Autodesk Inventor part; units mm, degrees
ref_plane "YZ Plane" through (0, 0, 0) normal (1, 0, 0) x (0, 1, 0)
ref_plane "XZ Plane" through (0, 0, 0) normal (0, 1, 0) x (-1, 0, 0)
ref_plane "XY Plane" through (0, 0, 0) normal (0, 0, 1) x (1, 0, 0)
sketch "Sketch1" plane through (0, 0, 0) normal (0, 0, 1) x (1, 0, 0)
  line L0 (0, 0) -> (160, 0)
  line L1 (160, 0) -> (160, 140)
  line L2 (160, 140) -> (0, 140)
  line L3 (0, 140) -> (0, 0)
  dimension "d0" = 160
  dimension "d1" = 140
extrude "Extrusion1" add sketch "Sketch1" along normal blind 3
fillet "Fillet1" radius 5 4 edges at (160, 140, 1.5) (0, 140, 1.5) (0, 0, 1.5) (160, 0, 1.5)
sketch "Sketch2" plane through (0, 0, 3) normal (0, 0, 1) x (1, 0, 0)
  arc A0 (155, 0) -> (160, 5) centre (155, 5) ccw
  line L0 (160, 5) -> (160, 135)
  arc A1 (160, 135) -> (155, 140) centre (155, 135) ccw
  line L1 (155, 140) -> (5, 140)
  arc A2 (5, 140) -> (0, 135) centre (5, 135) ccw
  line L2 (0, 135) -> (0, 5)
  arc A3 (0, 5) -> (5, 0) centre (5, 5) ccw
  line L3 (5, 0) -> (155, 0)
  line L4 (0, 0) -> (12.5, 0)
  line L5 (12.5, 0) -> (12.5, 12.5)
  line L6 (12.5, 12.5) -> (0, 12.5)
  line L7 (0, 12.5) -> (0, 0)
  circle A4 centre (12.5, 12.5) radius 1.5
  line L8 (80, 0) -> (80, 5)
  line L9 (0, 70) -> (5, 70)
  circle A5 centre (147.5, 12.5) radius 1.5
  circle A6 centre (12.5, 127.5) radius 1.5
  circle A7 centre (147.5, 127.5) radius 1.5
  dimension "d5" = 12.5
  dimension "d6" = 12.5
  dimension "d7" = 3
  dimension "d8" = 5
  dimension "d9" = 5
extrude "Extrusion2" cut sketch "Sketch2" against normal through all contours A4 L6 L5 | L5 L6 A4 | A5 | A6 | A7
fillet "Fillet2" radius 3 8 edges at (1.4645, 138.5355, 0) (0, 70, 0) (1.4645, 1.4645, 0) (80, 0, 0) (158.5355, 1.4645, 0) (160, 70, 0) (158.5355, 138.5355, 0) (80, 140, 0)
sketch "Sketch3" plane through (0, 0, 0) normal (0, 0, -1) x (-1, 0, 0)
  line L0 (-155, 140) -> (-5, 140)
  line L1 (-5, 0) -> (-155, 0)
  line L2 (-160, 5) -> (-160, 135)
  line L3 (0, 135) -> (0, 5)
  line L4 (-80, 0) -> (-80, 58)
  line L5 (-80, 58) -> (-115.5, 58)
  line L6 (-115.5, 58) -> (-115.5, 82)
  line L7 (-115.5, 82) -> (-80, 82)
  line L8 (-80, 82) -> (-80, 58)
  line L9 (-80, 58) -> (-44.5, 58)
  line L10 (-44.5, 58) -> (-44.5, 82)
  line L11 (-44.5, 82) -> (-80, 82)
  point P0 (0, 0)
  dimension "d13" = 58
  dimension "d14" = 35.5
  dimension "d15" = 24
extrude "Extrusion3" cut sketch "Sketch3" against normal blind 10
sketch "Sketch4" plane through (0, 0, 0) normal (0, 0, -1) x (-1, 0, 0)
  line L0 (-44.5, 58) -> (-115.5, 58)
  line L1 (-115.5, 58) -> (-115.5, 82)
  line L2 (-115.5, 82) -> (-44.5, 82)
  line L3 (-44.5, 82) -> (-44.5, 58)
  circle A0 centre (-12.5, 127.5) radius 1.5
  circle A1 centre (-147.5, 12.5) radius 1.5
  circle A2 centre (-147.5, 127.5) radius 1.5
  circle A3 centre (-12.5, 12.5) radius 1.5
  arc A4 (-3, 135) -> (-5, 137) centre (-5, 135) ccw
  line L4 (-155, 137) -> (-5, 137)
  arc A5 (-155, 137) -> (-157, 135) centre (-155, 135) ccw
  line L5 (-157, 5) -> (-157, 135)
  arc A6 (-157, 5) -> (-155, 3) centre (-155, 5) ccw
  line L6 (-5, 3) -> (-155, 3)
  arc A7 (-5, 3) -> (-3, 5) centre (-5, 5) ccw
  line L7 (-3, 135) -> (-3, 5)
  line L8 (-120.15, 87.8) -> (-40.15, 87.8)
  line L9 (-40.15, 51.8) -> (-120.15, 51.8)
  line L10 (-40.15, 51.8) -> (-40.15, 87.8)
  line L11 (-120.15, 51.8) -> (-120.15, 87.8)
  line L12 (-40.15, 51.8) -> (-42.65, 51.8)
  line L13 (-42.65, 51.8) -> (-42.65, 54.045)
  line L14 (-42.65, 54.045) -> (-40.15, 54.045)
  line L15 (-40.15, 54.045) -> (-40.15, 51.8)
  line L16 (-80.15, 51.8) -> (-80.15, 56.8)
  circle A8 centre (-42.65, 54.045) radius 1.5
  circle A9 centre (-117.65, 54.045) radius 1.5
  line L17 (-40.15, 87.8) -> (-42.616, 87.8)
  line L18 (-42.616, 87.8) -> (-42.616, 85.045)
  line L19 (-42.616, 85.045) -> (-40.15, 85.045)
  line L20 (-40.15, 85.045) -> (-40.15, 87.8)
  circle A10 centre (-42.616, 85.045) radius 1.5
  circle A11 centre (-117.684, 85.045) radius 1.5
  point P0 (0, 0)
  dimension "d18" = 5.8
  dimension "d19" = 6.2
  dimension "d20" = 4.35
  dimension "d21" = 4.65
  dimension "d22" = 2.5
  dimension "d23" = 2.245
  dimension "d24" = 5
  dimension "d25" = 3
  dimension "d26" = 2.466
  dimension "d27" = 2.755
  dimension "d28" = 3
extrude "Extrusion4" cut sketch "Sketch4" against normal blind 10 contours A10 L19 L18 | L18 L19 A10 | A8 L14 L13 | L13 L14 A8 | A9 | A11
properties part number "TutupBox"
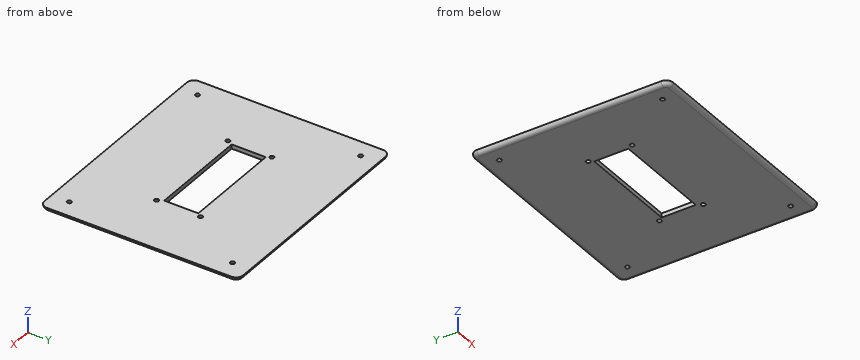
Can you work these out from the model? Positions are in its coordinate system, mm. Give positions to 0.01 mm unless a question says otherwise; leave off trailing zeros. Return JSON: item names as keys, results as strings.
1. If I drill on line 1 (X direction, y = 127.5, z = 1.95); line 2 (X direction, y = 127.5, z = 2.45); line 3 (Y direction, x = 147.5, z = 1.15), over which ranges is the centre line in solid material (lowest first)?
Output values:
{"line 1": "x = 0.19 to 11, 14 to 146, 149 to 159.81", "line 2": "x = 0.05 to 11, 14 to 146, 149 to 159.95", "line 3": "y = 0.64 to 11, 14 to 126, 129 to 139.36"}
2. I want a section at C-C on z = 2. Give the number of separate pieces and of enclosed holes in the cut face, and give its area (3 significant figures).
Output values:
{"separate pieces": "1", "enclosed holes": "9", "area": "20,500 mm²"}
3. I'm going to push flat-ended pins straight in: pin 1 Ø2.5 at (x, y) = (12.5, 12.5) entering from +Z; pin 2 Ø1.5 at (x, z) = (87.5, 2) entering from +Y; pin 3 Ø1 at (y, z) = (27, 0.5) entering from -X. Where does each tip first touch, or does it pass through?
Output values:
{"pin 1": "passes through", "pin 2": "stops at y = 139.99", "pin 3": "stops at x = 0.76"}
